The drawing under review shows one solid part. Ordinate dimensions are in mm from its lowest x, y, z. A direction names the side the tool comes from. Give positions to 0.01 mm unless a question says otherwise; leave off trailing zeros. Order: outer loops, then holes, each group sorted by start corner. A loop starts at its lowest first (then second) coordinate and runs counter-clockwise, first axis right, second up. Notation, with made-up numbers: (-23, 72) -> (-6, 72) arc R24 cw to (-6, 108) -> close; hole circle Ø11 at (-32.75, 39). An arc over 180 degrees is marked (long way). Return JSON: item names as keys, results as strings. Group by question number.
1) Insertion check: P1, Ø10, axis at x = 17, z = 27, coming from the +Y side; P2, Ø10, axis at x = 10.5, y = 19, coming from the +Z side; P3, Ø12, axis at x = 12, z = 7, coming from the +Y side. Each pin has a flat end and moves straight along its axis. Give the tip position at first contact, or say it passes through.
2) Add section A-A (z = 9). Give the boundary of the cut face in (x, y), then the cut area to 3 significant figures.
3) To check wall thickness, follow line 1 along X through (y, z) = (1.95, 9); line 2 along Y through (x, z) = (10, 2.2); line 3 along Y through (x, z) = (5.5, 24). State the ranges of each line that lie inside material, in increasing order.
4) Add section B-B (x = 10). Give the boundary of the cut face in (y, z).
5) Add section C-C (y = 17.5). Give the boundary of the cut face in (x, z), then the cut area to 3 significant figures.
6) Add section D-D (x = 4). Give the boundary of the cut face in (y, z).
7) The part is to be moulded in two halves that separate along X. For the marked faces 1, 2 and 3, say which applies: released by +X, released by -X, zero draft, split by the parting line, or undercut.
8) For the marked faces 4 and 5, list the 3-axis set-ups (+Z, -Z, +X, -X, +Y, -Y) from which the entire face can be reached by the end or side of a thin tool; tool diameter is ignored.
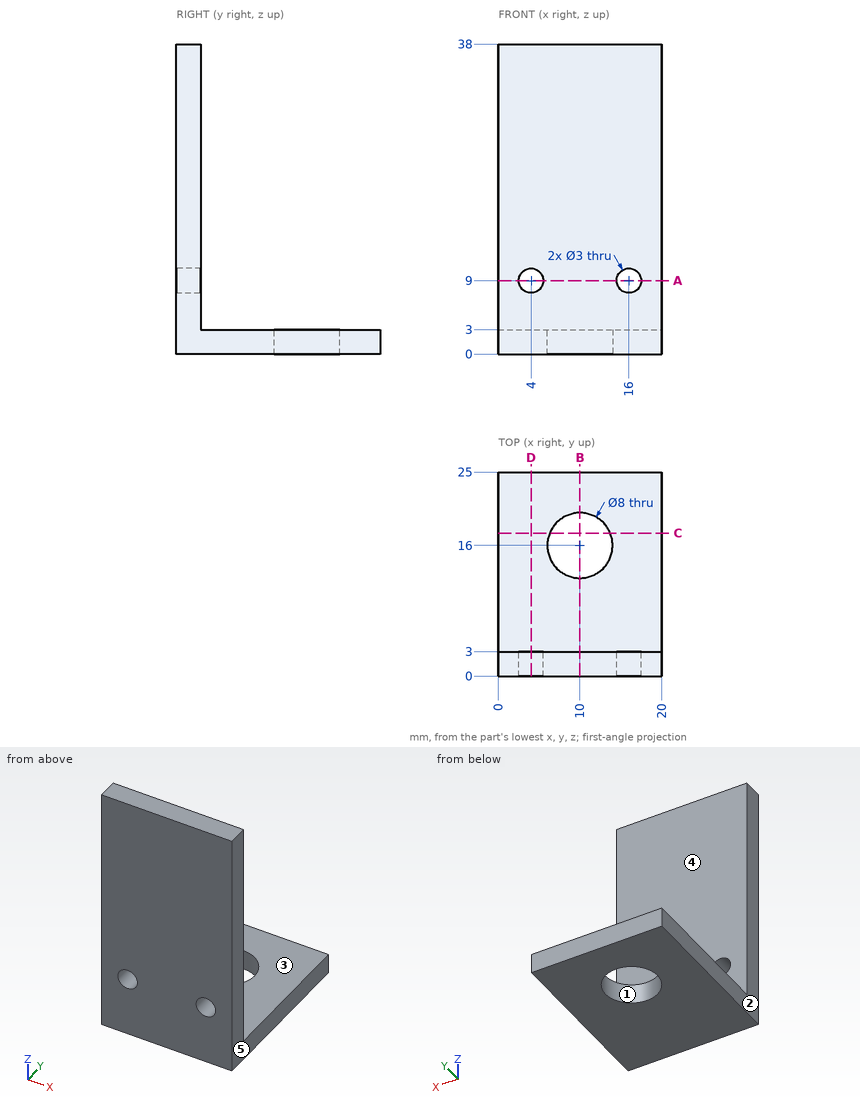
Evaluation:
{
 "1": {"P1": "y = 3", "P2": "z = 3", "P3": "y = 25"},
 "2": {"outline": "(0, 0) -> (2.5, 0) -> (2.5, 3) -> (0, 3) -> close; (5.5, 0) -> (14.5, 0) -> (14.5, 3) -> (5.5, 3) -> close; (17.5, 0) -> (20, 0) -> (20, 3) -> (17.5, 3) -> close", "area": "42.0 mm^2"},
 "3": {"line 1": "0 to 2.5, 5.5 to 14.5, 17.5 to 20", "line 2": "0 to 12, 20 to 25", "line 3": "0 to 3"},
 "4": {"outline": "(0, 0) -> (12, 0) -> (12, 3) -> (3, 3) -> (3, 38) -> (0, 38) -> close; (20, 0) -> (25, 0) -> (25, 3) -> (20, 3) -> close"},
 "5": {"outline": "(0, 0) -> (6.29, 0) -> (6.29, 3) -> (0, 3) -> close; (13.71, 0) -> (20, 0) -> (20, 3) -> (13.71, 3) -> close", "area": "37.8 mm^2"},
 "6": {"outline": "(0, 0) -> (25, 0) -> (25, 3) -> (3, 3) -> (3, 7.5) -> (0, 7.5) -> close; (0, 10.5) -> (3, 10.5) -> (3, 38) -> (0, 38) -> close"},
 "7": {"face 1": "undercut", "face 2": "released by -X", "face 3": "zero draft"},
 "8": {"face 4": "+Z, +X, -X, +Y", "face 5": "+Z, -Z, +X, +Y, -Y"}
}
